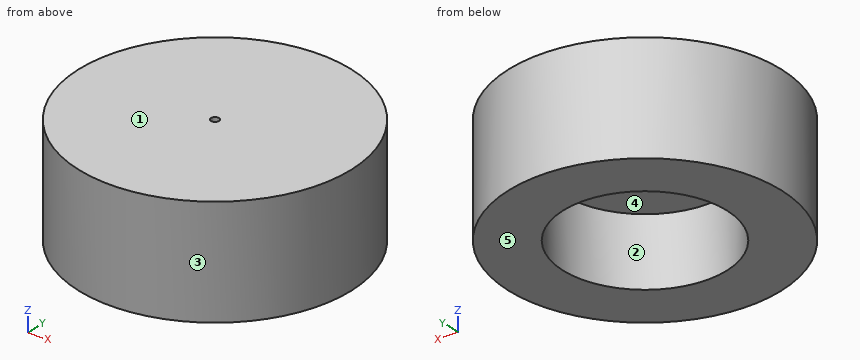
from build123d import *

# Parameters (mm, degrees)
SKETCH1_R           = 50
BOSS_EXTRUDE1_DEPTH = 40
SKETCH2_R           = 30
CUT_EXTRUDE1_DEPTH  = 25
CUT_EXTRUDE2_DEPTH  = 5
SKETCH5_R           = 1.5
CUT_EXTRUDE3_DEPTH  = 40


with BuildPart() as part:
    # Sketch1 → Boss-Extrude1 (new body)
    with BuildSketch(Plane.XY):
        Circle(SKETCH1_R)
    extrude(amount=BOSS_EXTRUDE1_DEPTH)

    # Sketch2 → Cut-Extrude1 (cut)
    with BuildSketch(Plane(origin=(0, 0, 0), x_dir=(-1, 0, 0), z_dir=(0, 0, -1))):
        Circle(SKETCH2_R)
    extrude(amount=-CUT_EXTRUDE1_DEPTH, mode=Mode.SUBTRACT)

    # Sketch3 → Cut-Extrude2 (cut)
    with BuildSketch(Plane(origin=(0, 0, 25), x_dir=(-1, 0, 0), z_dir=(0, 0, -1))):
        Polygon((4.082774554, -4.396697846), (5.849039304, 1.337437558), (1.76626475, 5.734135404), (-4.082774554, 4.396697846), (-5.849039304, -1.337437558), (-1.76626475, -5.734135404), align=None)
    extrude(amount=-CUT_EXTRUDE2_DEPTH, mode=Mode.SUBTRACT)

    # Sketch5 → Cut-Extrude3 (cut)
    with BuildSketch(Plane.XY.offset(40)):
        Circle(SKETCH5_R)
    extrude(amount=-CUT_EXTRUDE3_DEPTH, mode=Mode.SUBTRACT)


solid = part.part
Source: CAD feature listing. Evaluate the final solid. Frame: model axes, mm. Face numbers are marked on the shaded views. A direction names the side the tool comes from. Round coordinates to 2 decimals unless told otherwise and drop trailing zeros. Loops run counter-clockwise (first coordinate to the right, second up) from the corner with the lowest first, then second, coordinate; pieces in that order, holes last. Notation, with made-up numbers: M 68,87 L 72,87 A15 cw 72,114 Z; hole C 68,48.5 d3. An arc over 180 degrees is marked long. Return JSON: item names as keys, results as strings. Group by question number.
1. Section query A-A on x = 0. Output: boundary loops of the cut face in (y, z), and give its area (3 significant figures).
2. Reachability of the marked faces 4 and 5 from +Z, -Z, +X, -X, +Y, -Y: full face, straight path, thin tool, end or side. Return the list, or none.
3. Section query C-C on y = 0. Output: boundary loops of the cut face in (x, z), and give its area (3 significant figures).
4. Section query B-B on z = 15. Output: boundary loops of the cut face in (x, y), and give its area (3 significant figures).
5. Mould query, pull axis Y, two halves, no side actions, for the marked faces 1, 2 and 3. Classes: released by +Y, released by -Y, zero draft, split by the parting line, or undercut.
6. Section query D-D on x = 17.5. Output: boundary loops of the cut face in (y, z), and give its area (3 significant figures).
7. Pin query (flat end, axial travel): pin 1 (4 mm diameter, centred on x = 23, y = 3, fed in from -Z); pin 2 (1 mm diameter, centred on x = 18.5, z = 16.5, fed in from +Y); pin 3 (6 mm diameter, centred on y = 22.5, z = 14, fed in from +X). Return the tip coordinate at first contact, or that it passes through.
8. Material intervals for line 1 along Y through (x, z) = (0, 13.5); line 2 along Y through (x, z) = (-8, 19); line 3 along X through (y, z) = (9.5, 18.5), sorted ascending. Write a range as from..to.
Checks:
{
 "1": {"outline": "M -50,0 L -30,0 L -30,25 L -5.33,25 L -5.33,30 L -1.5,30 L -1.5,40 L -50,40 Z; M 1.5,30 L 5.33,30 L 5.33,25 L 30,25 L 30,0 L 50,0 L 50,40 L 1.5,40 Z", "area": "2,420 mm²"},
 "2": {"face 4": "-Z", "face 5": "-Z, +X, -X, +Y, -Y"},
 "3": {"outline": "M -50,0 L -30,0 L -30,25 L -5.44,25 L -5.44,30 L -1.5,30 L -1.5,40 L -50,40 Z; M 1.5,30 L 5.44,30 L 5.44,25 L 30,25 L 30,0 L 50,0 L 50,40 L 1.5,40 Z", "area": "2,420 mm²"},
 "4": {"outline": "C 0,0 d100; hole C 0,0 d60", "area": "5,030 mm²"},
 "5": {"face 1": "zero draft", "face 2": "undercut", "face 3": "split by the parting line"},
 "6": {"outline": "M -46.84,0 L -24.37,0 L -24.37,25 L 24.37,25 L 24.37,0 L 46.84,0 L 46.84,40 L -46.84,40 Z", "area": "2,530 mm²"},
 "7": {"pin 1": "stops at z = 25", "pin 2": "stops at y = 46.65", "pin 3": "stops at x = 46.04"},
 "8": {"line 1": "y = -50..-30, 30..50", "line 2": "y = -49.36..-28.91, 28.91..49.36", "line 3": "x = -49.09..-28.46, 28.46..49.09"}
}
